Here's how the part is built. I have some questions about the finished solid (model axes, mm). A direction names the side the tool comes from. Round coordinates to 2 decimals unless told otherwise and drop trailing zeros. Write each loop counter-clockwise with the first axis right and the second up, starting at its lowest first coordinate (ties: lowest second). Pieces come first, ordered by that corner, then holes. Notation, with made-up numbers: (20, 67) -> (76, 67) arc R28 ccw to (76, 94) -> close; hole circle Ø9 at (81, -9). An arc over 180 degrees is marked (long way). Answer in a Markdown table with one row per item. Add a question column.
from build123d import *

# Parameters (mm, degrees)
SKETCH1_R   = 12.7
SKETCH1_R_2 = 10.6807


with BuildPart() as part:
    # Sweep7: sweep along a path in Sketch15
    with BuildLine(Plane(origin=(0, 0, 0), x_dir=(1, 0, 0), z_dir=(0, 1, 0))) as sweep7_path:
        Line((0, 0), (0, 12.7))
        ThreePointArc((0, 12.7), (7.439487758, 30.660512242), (25.4, 38.1))
        Line((25.4, 38.1), (38.1, 38.1))
    # Sketch1 → Sweep7 (sweep)
    with BuildSketch(Plane.XY):
        Circle(SKETCH1_R)
        Circle(SKETCH1_R_2, mode=Mode.SUBTRACT)
    sweep(path=sweep7_path.line)


solid = part.part
Item 1: If we mould it in two halves opening along X, with no side actions, what happens to faces 3 (the cylindrical face through (9.866, 4.091, -6.439)), 4 (the cylindrical face through (-2.75, 12.4, -6.44)), 5 (the flat face through (38.1, -9, -31))? For each: pulls with the +X half, pulls with the -X half, needs draft (parallel to the pull), parting line crosses it, or undercut.
Item 2: On a 3-axis mill with a long thin cutter (end or side, diameter ignored), from which of +Z, -Z, +X, -X, +Y, -Y can I reach the whole of each face in a straight line? I mean faces 1 (the flat face through (-7, 9, 0)), 2 (the cylindrical face through (31.84, -0.47, -48.77)). Say none if no direction works.
Item 3: I need wall thicknesses on line 1 along Y through (x, z) = (28, -38); line 2 along Z through (x, y) = (34.75, 0). Which ranges of each line are inside material? Lowest first, please. Write a range as from..to.
Item 4: If we section it at B-B on x = 31: Please give me the cut outline in (y, z).
Item 5: If we section it at A-A on y = 0: Please give me the cut outline in (x, z).
Item 6: If we section it at C-C on y = 9.5: Please give me the cut outline in (x, z), then the cut area to 3 significant figures.
Item 7: For P1, Ø12, axis at y = -6, z = -26, coming from the -X side; P2, Ø12, axis at x = 10.5, z = -12, coming from the -Y side; P3, Ø12, axis at x = 23.5, y = 0.5, coming from the +Z side, each with a flat end and sliding along its axis, tell me the tip position at first contact or that it passes through.
Results list:
| question | item | result |
|---|---|---|
| 1 | face 3 | undercut |
| 1 | face 4 | parting line crosses it |
| 1 | face 5 | pulls with the +X half |
| 2 | face 1 | +Z, +X, -X, +Y, -Y |
| 2 | face 2 | +X |
| 3 | line 1 | -12.7..-10.68, 10.68..12.7 |
| 3 | line 2 | -50.8..-48.78, -27.42..-25.4 |
| 4 | outline | circle Ø25.4 at (0, -38.1); hole circle Ø21.36 at (0, -38.1) |
| 5 | outline | (-12.7, -12.7) arc R38.1 ccw to (25.4, -50.8) -> (38.1, -50.8) -> (38.1, -48.78) -> (25.4, -48.78) arc R36.08 cw to (-10.68, -12.7) -> (-10.68, 0) -> (-12.7, 0) -> close; (10.68, -12.7) arc R14.72 ccw to (25.4, -27.42) -> (38.1, -27.42) -> (38.1, -25.4) -> (25.4, -25.4) arc R12.7 cw to (12.7, -12.7) -> (12.7, 0) -> (10.68, 0) -> close |
| 6 | outline | (-8.43, -12.7) arc R33.83 ccw to (25.4, -46.53) -> (38.1, -46.53) -> (38.1, -42.98) -> (25.4, -42.98) arc R30.28 cw to (-4.88, -12.7) -> (-4.88, 0) -> (-8.43, 0) -> close; (4.88, -12.7) arc R20.52 ccw to (25.4, -33.22) -> (38.1, -33.22) -> (38.1, -29.67) -> (25.4, -29.67) arc R16.97 cw to (8.43, -12.7) -> (8.43, 0) -> (4.88, 0) -> close |
| 6 | area | 463 mm² |
| 7 | P1 | x = -11.51 |
| 7 | P2 | y = -11.88 |
| 7 | P3 | z = -22.65 |
